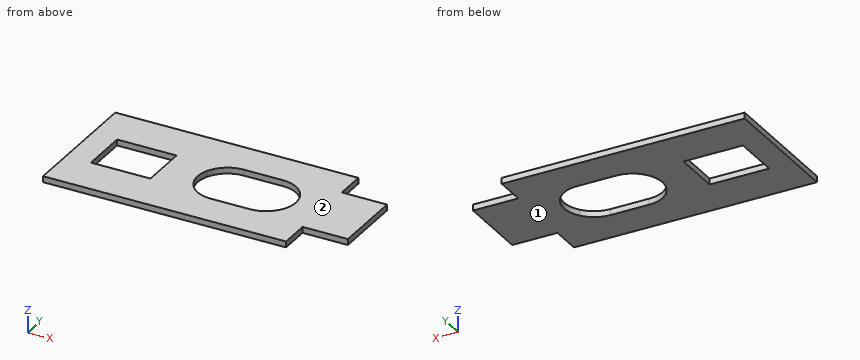
from build123d import *

# Parameters (mm, degrees)
BOSS_EXTRUDE2_DEPTH = 0.762


with BuildPart() as part:
    # Sketch1 → Boss-Extrude2 (new body)
    with BuildSketch(Plane.XY.offset(0.762)):
        with BuildLine():
            Line((21.595288772, -19.1309), (-9.44245, -19.1309))
            Line((-9.44245, -19.1309), (-9.44245, -20.7184))
            Line((-9.44245, -20.7184), (14.94155, -20.7184))
            ThreePointArc((14.94155, -20.7184), (16.737601224, -21.462348776), (17.48155, -23.2584))
            Line((17.48155, -23.2584), (17.48155, -25.2015))
            ThreePointArc((17.48155, -25.2015), (18.24355, -27.4875), (17.48155, -29.7735))
            Line((17.48155, -29.7735), (17.48155, -31.7166))
            ThreePointArc((17.48155, -31.7166), (16.737601224, -33.512651224), (14.94155, -34.2566))
            Line((14.94155, -34.2566), (-9.44245, -34.2566))
            Line((-9.44245, -34.2566), (-9.44245, -35.8441))
            Line((-9.44245, -35.8441), (21.595288772, -35.8441))
            Line((21.595288772, -35.8441), (21.595288772, -32.01505))
            Line((21.595288772, -32.01505), (27.373788772, -32.01505))
            Line((27.373788772, -32.01505), (27.373788772, -22.95995))
            Line((27.373788772, -22.95995), (26.103788772, -22.95995))
            Line((26.103788772, -22.95995), (21.595288772, -22.95995))
            Line((21.595288772, -22.95995), (21.595288772, -19.1309))
        make_face()
        with BuildLine():
            Line((14.94155, -20.7184), (-9.44245, -20.7184))
            Line((-9.44245, -20.7184), (-9.44245, -34.2566))
            Line((-9.44245, -34.2566), (14.94155, -34.2566))
            ThreePointArc((14.94155, -34.2566), (16.737601224, -33.512651224), (17.48155, -31.7166))
            Line((17.48155, -31.7166), (17.48155, -29.7735))
            ThreePointArc((17.48155, -29.7735), (16.137433799, -30.895267598), (14.43355, -31.2975))
            Line((14.43355, -31.2975), (9.49325, -31.2975))
            ThreePointArc((9.49325, -31.2975), (7.419008087, -30.683375543), (6.01345, -29.03898057))
            Line((6.01345, -29.03898057), (6.01345, -30.44025))
            Line((6.01345, -30.44025), (1.32715, -30.44025))
            Line((1.32715, -30.44025), (1.32715, -30.51645))
            Line((1.32715, -30.51645), (-6.26745, -30.51645))
            Line((-6.26745, -30.51645), (-6.26745, -24.45855))
            Line((-6.26745, -24.45855), (1.32715, -24.45855))
            Line((1.32715, -24.45855), (1.32715, -24.53475))
            Line((1.32715, -24.53475), (6.01345, -24.53475))
            Line((6.01345, -24.53475), (6.01345, -25.93601943))
            ThreePointArc((6.01345, -25.93601943), (7.419008087, -24.291624457), (9.49325, -23.6775))
            Line((9.49325, -23.6775), (14.43355, -23.6775))
            ThreePointArc((14.43355, -23.6775), (16.137433799, -24.079732402), (17.48155, -25.2015))
            Line((17.48155, -25.2015), (17.48155, -23.2584))
            ThreePointArc((17.48155, -23.2584), (16.737601224, -21.462348776), (14.94155, -20.7184))
        make_face()
        with BuildLine():
            ThreePointArc((6.01345, -29.03898057), (5.68325, -27.4875), (6.01345, -25.93601943))
            Line((6.01345, -25.93601943), (6.01345, -24.53475))
            Line((6.01345, -24.53475), (1.32715, -24.53475))
            Line((1.32715, -24.53475), (1.32715, -30.44025))
            Line((1.32715, -30.44025), (6.01345, -30.44025))
            Line((6.01345, -30.44025), (6.01345, -29.03898057))
        make_face()
    extrude(amount=BOSS_EXTRUDE2_DEPTH)


solid = part.part
Read the model definition and answer for the solid it produces. Units are mm, in the model's axes. Face numbers are marked on the shaded views. Coordinates: 2 decimals unless noted, no trailing zeros. Write each loop counter-clockwise with the first axis right and the second up, starting at its lowest first coordinate (ties: lowest second). Pieces come first, ordered by that corner, then holes. Notation, with made-up numbers: (8, 61.5) -> (27, 61.5) arc R21 ccw to (27, 100.5) -> close; hole circle Ø5 at (71.5, -8). An arc over 180 degrees is marked (long way). Return JSON: item names as keys, results as strings.
(1) The part is cut by section B-B on x = -1. Give the vertices of the cut face in (y, z), then the cut area to 3 significant figures.
Answers below:
{"outline": "(-35.84, 0.76) -> (-30.52, 0.76) -> (-30.52, 1.52) -> (-35.84, 1.52) -> close; (-24.46, 0.76) -> (-19.13, 0.76) -> (-19.13, 1.52) -> (-24.46, 1.52) -> close", "area": "8.12 mm^2"}
(2) The part is cut by section D-D on y = -33. Give the vertices of the cut face in (x, z), then the cut area to 3 significant figures.
Answers below:
{"outline": "(-9.44, 0.76) -> (21.6, 0.76) -> (21.6, 1.52) -> (-9.44, 1.52) -> close", "area": "23.7 mm^2"}
(3) Consider line 1 along X through (y, z) = (-29.5, 1.25); line 2 along X through (y, z) = (-26.25, 1.1); line 3 along Y through (x, z) = (-6, 1.15). Determine where each line is inside the solid, lowest interval first. Write a range as from..to.
Answers below:
{"line 1": "-9.44..-6.27, 1.33..6.26, 17.67..27.37", "line 2": "-9.44..-6.27, 1.33..5.89, 18.04..27.37", "line 3": "-35.84..-30.52, -24.46..-19.13"}
(4) The part is cut by section C-C on y = -27. Give the vertices of the cut face in (x, z), then the cut area to 3 significant figures.
Answers below:
{"outline": "(-9.44, 0.76) -> (-6.27, 0.76) -> (-6.27, 1.52) -> (-9.44, 1.52) -> close; (1.33, 0.76) -> (5.71, 0.76) -> (5.71, 1.52) -> (1.33, 1.52) -> close; (18.21, 0.76) -> (27.37, 0.76) -> (27.37, 1.52) -> (18.21, 1.52) -> close", "area": "12.7 mm^2"}
(5) For a pull along Z with two mould halves and no side action, classify the marked faces 1 and 2 as pulls with the +Z half, pulls with the -Z half, needs draft (parallel to the pull), parting line crosses it, or undercut.
Answers below:
{"face 1": "pulls with the -Z half", "face 2": "pulls with the +Z half"}
(6) The part is cut by section A-A on z = 1. Give the vertices of the cut face in (x, y).
Answers below:
{"outline": "(-9.44, -35.84) -> (21.6, -35.84) -> (21.6, -32.02) -> (27.37, -32.02) -> (27.37, -22.96) -> (21.6, -22.96) -> (21.6, -19.13) -> (-9.44, -19.13) -> close; hole (-6.27, -30.52) -> (1.33, -30.52) -> (1.33, -24.46) -> (-6.27, -24.46) -> close; hole (9.49, -31.3) -> (14.43, -31.3) arc R3.81 ccw to (14.43, -23.68) -> (9.49, -23.68) arc R3.81 ccw to start"}
